```python
from build123d import *

# Parameters (mm, degrees)
F0_R     = 6
F1_DEPTH = 46
F2_W     = 36
F2_H     = 28.489591
F3_DEPTH = 25


with BuildPart() as f1:
    # F0 (on Front) → F1 (new body)
    with BuildSketch(Plane.XZ):
        with BuildLine():
            Line((5, -45), (5, 0))
            Line((5, 0), (15, 0))
            Line((15, 0), (15, 22))
            Line((15, 22), (9, 22))
            Line((9, 22), (9, 6))
            Line((9, 6), (0, 6))
            Line((0, 6), (-9, 6))
            Line((-9, 6), (-9, 22))
            Line((-9, 22), (-15, 22))
            Line((-15, 22), (-15, 0))
            Line((-15, 0), (-5, 0))
            Line((-5, 0), (-5, -67))
            Line((-5, -67), (5, -67))
            Line((5, -67), (13, -67))
            ThreePointArc((13, -67), (24, -56), (13, -45))
            Line((13, -45), (5, -45))
        make_face()
        with Locations((13, -56)):
            Circle(F0_R, mode=Mode.SUBTRACT)
    extrude(amount=F1_DEPTH)


with BuildPart() as f3:
    # F2 (on face) → F3 (new body)
    with BuildSketch(Plane.YZ.offset(5)):
        with Locations((-23, -59.244795)):
            Rectangle(F2_W, F2_H)
    extrude(amount=F3_DEPTH)


with BuildPart() as f1_1:
    add(f1.part)

    # F4: cut F3
    add(f3.part, mode=Mode.SUBTRACT)


solid = f1_1.part
```
Can you work these out from the model? Positions are in its coordinate system, mm. A direction names the side the tool comes from. Give positions to 0.01 mm unless a question says otherwise; leave off trailing zeros. Order: outer loops, then holes, each group sorted by start corner. A loop starts at its lowest first (then second) coordinate and runs counter-clockwise, first axis right, second up. Notation, with made-up numbers: (73.5, 3) - (85.5, 3) arc R18 cw to (85.5, 8) - close; hole circle Ø3 at (-5, 9.25). An arc over 180 degrees is marked (long way). Use a Markdown table: item, result. Add a question column.
Q1. If we section it at D-D on y = -32: Write out the boundary of the cut face in (x, z), plus the area to 3 significant figures.
Q2. If we section it at A-A on z = 15: Write out the boundary of the cut face in (x, y).
Q3. If we section it at B-B on x = 12: Write out the boundary of the cut face in (y, z), plus the area to 3 significant figures.
Q4. If we section it at C-C on z = -56: Write out the boundary of the cut face in (x, y).
Q5. I'm going to push flat-ended pins straight in: pin 1 (5 mm diameter, centred on x = -8.5, y = -8.5, fed in from -Z); pin 2 (14 mm diameter, centred on y = -15.5, z = -23.5, fed in from +X); pin 3 (5.5 mm diameter, centred on x = -2, y = -22, fed in from +Z). Where does each tip first touch, or does it pass through?
Q6. If we mould it in two halves opening along Y, with no side actions, what happens to faces 1 (the flat face through (19, -5, -54)), 2 (the flat face through (-5, -23, -33)), 3 (the flat face through (4, -46, -32))? For each: released by +Y, released by -Y, zero draft, split by the parting line, or undercut.
Q7. Please list where these lines run through material, in increasing order: line 1 along Z through (x, y) = (13, -2.95); line 2 along Y through (x, z) = (14, -62.5); line 3 along X through (y, z) = (-3, -56).
Q8. On a 3-axis mill with a long thin cutter (end or side, diameter ignored), from which of +Z, -Z, +X, -X, +Y, -Y can I reach the whole of each face in a straight line? I mean faces 4 (the flat face through (19, -41, -54)), 5 (the flat face through (10, -23, 0)), 6 (the flat face through (9, -23, 14)). Say none if no direction works.
Answers follow:
| question | item | result |
|---|---|---|
| 1 | outline | (-15, 0) - (-5, 0) - (-5, -67) - (5, -67) - (5, 0) - (15, 0) - (15, 22) - (9, 22) - (9, 6) - (-9, 6) - (-9, 22) - (-15, 22) - close |
| 1 | area | 1,040 mm^2 |
| 2 | outline | (-15, -46) - (-9, -46) - (-9, 0) - (-15, 0) - close; (9, -46) - (15, -46) - (15, 0) - (9, 0) - close |
| 3 | outline | (-46, -67) - (-41, -67) - (-41, -61.92) - (-46, -61.92) - close; (-46, -50.08) - (-41, -50.08) - (-41, -45) - (-46, -45) - close; (-46, 0) - (0, 0) - (0, 22) - (-46, 22) - close; (-5, -67) - (0, -67) - (0, -61.92) - (-5, -61.92) - close; (-5, -50.08) - (0, -50.08) - (0, -45) - (-5, -45) - close |
| 3 | area | 1,110 mm^2 |
| 4 | outline | (-5, -46) - (7, -46) - (7, -41) - (5, -41) - (5, -5) - (7, -5) - (7, 0) - (-5, 0) - close; (19, -46) - (24, -46) - (24, -41) - (19, -41) - close; (19, -5) - (24, -5) - (24, 0) - (19, 0) - close |
| 5 | pin 1 | stops at z = 0 |
| 5 | pin 2 | stops at x = 5 |
| 5 | pin 3 | stops at z = 6 |
| 6 | face 1 | undercut |
| 6 | face 2 | zero draft |
| 6 | face 3 | released by -Y |
| 7 | line 1 | z = -67 to -62, -50 to -45, 0 to 22 |
| 7 | line 2 | y = -46 to -41, -5 to 0 |
| 7 | line 3 | x = -5 to 7, 19 to 24 |
| 8 | face 4 | -Z, +X |
| 8 | face 5 | +X, +Y, -Y |
| 8 | face 6 | +Z, +Y, -Y |
